from build123d import *

# Parameters (mm, degrees)
SKETCH_W     = 12
SKETCH_H     = 10
SKETCH_R     = 1.2
PAD_DEPTH    = 6
SKETCH001_W  = 12
SKETCH001_H  = 4
PAD001_DEPTH = 45
SKETCH002_W  = 12
SKETCH002_H  = 14
PAD002_DEPTH = 4
SKETCH005_R  = 2.5
POCKET_DEPTH = 5


with BuildPart() as part:
    # Sketch → Pad (new body)
    with BuildSketch(Plane.XY):
        with Locations((-6, 5)):
            Rectangle(SKETCH_W, SKETCH_H)
        with Locations((-9, 7)):
            Circle(SKETCH_R, mode=Mode.SUBTRACT)
        with Locations((-3, 7)):
            Circle(SKETCH_R, mode=Mode.SUBTRACT)
    extrude(amount=PAD_DEPTH)

    # Sketch001 (on Face8 of Pad) → Pad001 (join)
    with BuildSketch(Plane.XY.offset(6)):
        with Locations((-6, 2)):
            Rectangle(SKETCH001_W, SKETCH001_H)
    extrude(amount=PAD001_DEPTH)

    # Sketch002 (on Face13 of Pad001) → Pad002 (join)
    with BuildSketch(Plane.XY.offset(51)):
        with Locations((-6, 7)):
            Rectangle(SKETCH002_W, SKETCH002_H)
    extrude(amount=PAD002_DEPTH)

    # Sketch005 (on Face18 of Pad002) → Pocket (cut)
    with BuildSketch(Plane.XY.offset(55)):
        with Locations((-6, 9)):
            Circle(SKETCH005_R)
    extrude(amount=-POCKET_DEPTH, mode=Mode.SUBTRACT)


solid = part.part
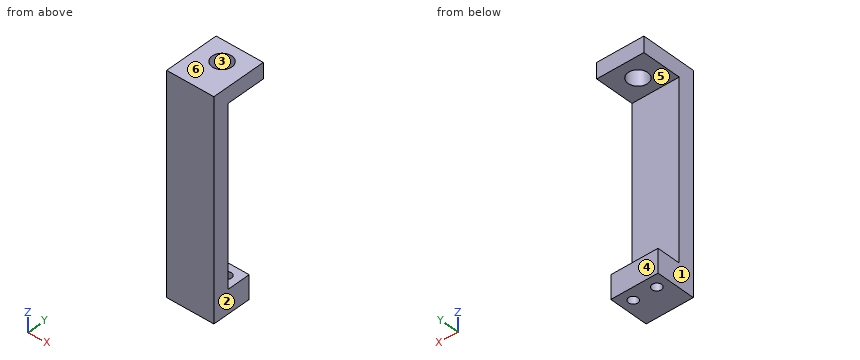
For this review, take the finished solid that the model builds, in its own axes (mm). Face numbers are marked on the shaded views. A direction names the side the tool comes from. Give positions to 0.01 mm unless a question says otherwise; leave off trailing zeros. Order: outer loops, then holes, each group sorted by start corner. A loop starts at its lowest first (then second) coordinate and runs counter-clockwise, first axis right, second up. Notation, with made-up numbers: (-2, -21.5) - (4, -21.5) arc R32 cw to (4, 15.5) - close; hole circle Ø6 at (87.25, 37). An arc over 180 degrees is marked (long way). Answer as a JSON object with one key per item and string values. Group by question number.
Item 1: Take a section at D-D on x = -11. Give the boundary of the cut face in (y, z), and give its area (3 significant figures).
Item 2: Take a section at A-A on x = -6. Give the boundary of the cut face in (y, z).
Item 3: Draft analysis for pull direction X (two halves, no side actions). For the marked faces 1, 2, 3 and 4, state which applies: pulls with the +X half, pulls with the -X half, needs draft (parallel to the pull), parting line crosses it, or undercut.
Item 4: Machinability: for the marked faces 5 and 6, which of the approach directions +Z, -Z, +X, -X, +Y, -Y give a long, thin tool a straight path to every point of the face, cutting with its end or side? Answer none if there is none.
Item 5: Wall thickness on line 1 along Z through (x, y) = (-1.25, 8.75); line 2 along Y through (x, z) = (-3, 4.45); line 3 along Y through (x, z) = (-6, 51.9): over which ranges is each line inside the solid? List them lowest first.
Item 6: Take a section at C-C on y = 9. Give the boundary of the cut face in (x, z).
Item 7: Take a section at B-B on y = 5. Give the boundary of the cut face in (x, z), and give its area (3 significant figures).
Item 8: Clearance check with flat-ended pins moving along their axes: pin 1 Ø3 at (x, z) = (-3, 14) entering from +Y; pin 2 Ø5 at (x, z) = (-7, 2) entering from +Y. State where each tip first meets the part, or that it passes through.
Reported:
{
 "1": {"outline": "(0, 0) - (10, 0) - (10, 6) - (4, 6) - (4, 51) - (14, 51) - (14, 55) - (0, 55) - close", "area": "296 mm^2"},
 "2": {"outline": "(0, 0) - (10, 0) - (10, 6) - (4, 6) - (4, 51) - (6.5, 51) - (6.5, 55) - (0, 55) - close; (11.5, 51) - (14, 51) - (14, 55) - (11.5, 55) - close"},
 "3": {"face 1": "pulls with the -X half", "face 2": "pulls with the +X half", "face 3": "undercut", "face 4": "needs draft"},
 "4": {"face 5": "+X, -X, +Y", "face 6": "+Z, +X, -X, +Y, -Y"},
 "5": {"line 1": "0 to 6, 51 to 55", "line 2": "0 to 5.8, 8.2 to 10", "line 3": "0 to 6.5, 11.5 to 14"},
 "6": {"outline": "(-12, 0) - (0, 0) - (0, 6) - (-12, 6) - close; (-12, 51) - (-8.5, 51) - (-8.5, 55) - (-12, 55) - close; (-3.5, 51) - (0, 51) - (0, 55) - (-3.5, 55) - close"},
 "7": {"outline": "(-12, 0) - (0, 0) - (0, 6) - (-12, 6) - close; (-12, 51) - (0, 51) - (0, 55) - (-12, 55) - close", "area": "120 mm^2"},
 "8": {"pin 1": "y = 4", "pin 2": "y = 10"}
}
